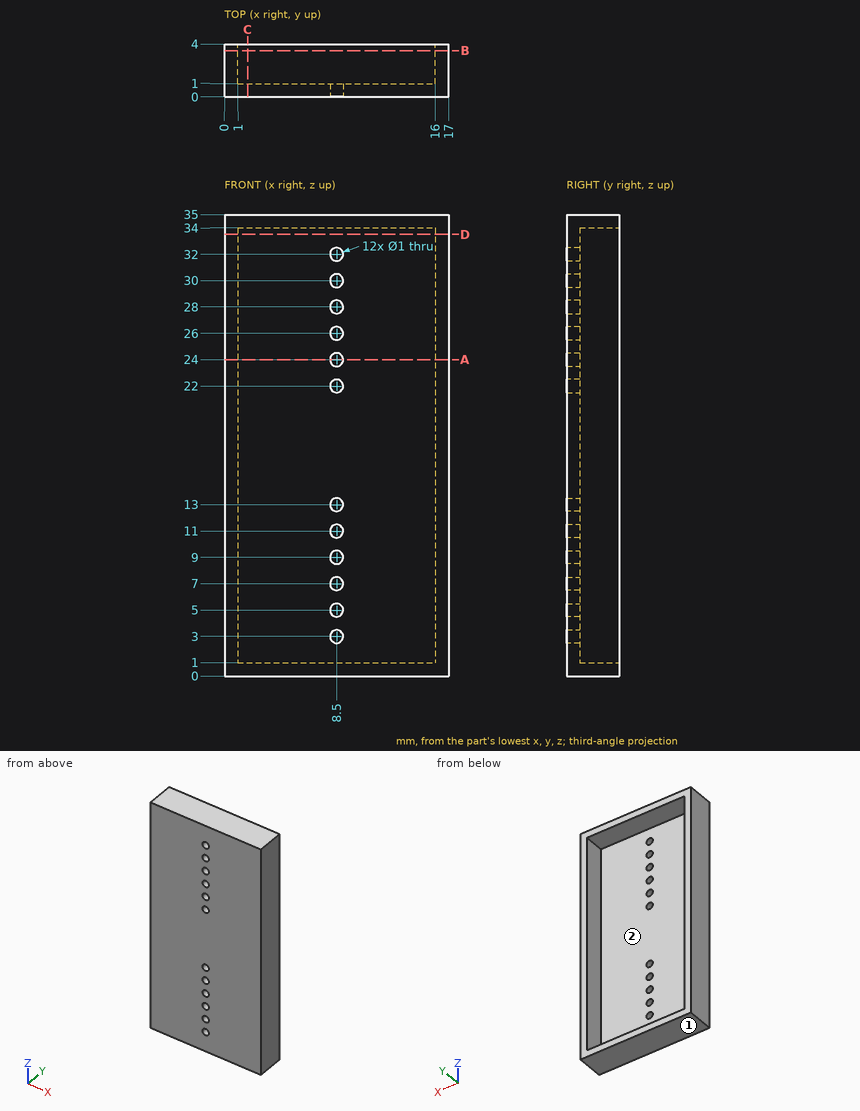
Design review of the part shown in the three views and the two pictorial views. Dimensions are in mm from the part's minimum x, y and z. A direction names the side the tool comes from. Give positions to 0.01 mm unless a question says otherwise; leave off trailing zeros. Write each loop counter-clockwise with the first axis right and the second up, starting at its lowest first coordinate (ties: lowest second). Pieces come first, ordered by that corner, then holes.
Item 1: Take a section at A-A (z = 24). Give the boundary of the cut face in (x, y).
Item 2: Take a section at C-C (x = 1.75). Give the boundary of the cut face in (y, z), and give its area (3 significant figures).
Item 3: Wall thickness on probe 1 along Z at (x, y) = (7, 1.9); probe 2 along X at (y, z) = (3.55, 14); probe 3 along X at (y, z) = (0.85, 3): over which ranges is each line inside the solid? List them lowest first.
Item 4: Take a section at D-D (z = 33.5). Give the boundary of the cut face in (x, y).
Item 5: Insertion check: P1, Ø1, axis at y = 3.5, z = 7.5, coming from the -X side. The pin has a flat end and moves straight along its axis. Give the tip position at first contact, or say it passes through.
Item 6: Take a section at B-B (y = 3.5). Give the boundary of the cut face in (x, z), and give its area (3 significant figures).
Item 7: Machinability: for the marked faces 1 and 2, which of the approach directions +Z, -Z, +X, -X, +Y, -Y give a long, thin tool a straight path to every point of the face, cutting with its end or side? Answer none if there is none.
Established:
1. outline: (0, 0) - (8, 0) - (8, 1) - (1, 1) - (1, 4) - (0, 4) - close; (9, 0) - (17, 0) - (17, 4) - (16, 4) - (16, 1) - (9, 1) - close
2. outline: (0, 0) - (4, 0) - (4, 1) - (1, 1) - (1, 34) - (4, 34) - (4, 35) - (0, 35) - close
2. area: 41.0 mm2
3. probe 1: z = 0 to 1, 34 to 35
3. probe 2: x = 0 to 1, 16 to 17
3. probe 3: x = 0 to 8, 9 to 17
4. outline: (0, 0) - (17, 0) - (17, 4) - (16, 4) - (16, 1) - (1, 1) - (1, 4) - (0, 4) - close
5. P1: stops at x = 0
6. outline: (0, 0) - (17, 0) - (17, 35) - (0, 35) - close; hole (1, 1) - (16, 1) - (16, 34) - (1, 34) - close
6. area: 100 mm2
7. face 1: -Z, +X, -X, +Y, -Y
7. face 2: +Y
